Autodesk Inventor part; units mm, degrees
ref_plane "YZ Plane" through (0, 0, 0) normal (1, 0, 0) x (0, 1, 0)
ref_plane "XZ Plane" through (0, 0, 0) normal (0, 1, 0) x (-1, 0, 0)
ref_plane "XY Plane" through (0, 0, 0) normal (0, 0, 1) x (1, 0, 0)
sketch "Sketch1" plane through (0, 0, 0) normal (1, 0, 0) x (0, 1, 0)
  line L0 (4.2484, 4.9473) -> (-21.1516, 4.9473)
  line L1 (-21.1516, 4.9473) -> (-21.1516, -20.4527)
  line L2 (-21.1516, -20.4527) -> (4.2484, -20.4527)
  line L3 (4.2484, -20.4527) -> (4.2484, 4.9473)
  line L4 (1.0734, 1.7723) -> (-17.9766, 1.7723)
  line L5 (-17.9766, 1.7723) -> (-17.9766, -17.2777)
  line L6 (-17.9766, -17.2777) -> (1.0734, -17.2777)
  line L7 (1.0734, -17.2777) -> (1.0734, 1.7723)
  point P0 (0, 0)
  dimension "d0" = 25.4
  dimension "d1" = 25.4
  dimension "d2" = 3.175
extrude "Extrusion1" add sketch "Sketch1" along normal blind 381
sketch "Sketch2" plane through (0, -21.1516, -20.4527) normal (0, 0, -1) x (-1, 0, 0)
  line L0 (0, 0) -> (0, 25.4) construction
  line L1 (0, 12.7) -> (-12.7, 12.7) construction
  line L2 (-12.7, 12.7) -> (-38.1, 12.7) construction
  line L3 (-381, 0) -> (-381, 25.4) construction
  line L4 (-381, 12.7) -> (-368.3, 12.7) construction
  line L5 (-368.3, 12.7) -> (-342.9, 12.7) construction
  circle A0 centre (-368.3, 12.7) radius 2.5797
  circle A1 centre (-342.9, 12.7) radius 2.5797
  circle A2 centre (-12.7, 12.7) radius 2.5797
  circle A3 centre (-38.1, 12.7) radius 2.5797
  point P0 (0, 21.1516)
  dimension "d5" = 12.7
  dimension "d6" = 25.4
  dimension "d7" = 12.7
  dimension "d8" = 25.4
  dimension "d9" = 5.1594
  dimension "d10" = 5.1594
  dimension "d11" = 5.1594
  dimension "d12" = 5.1594
extrude "Extrusion2" cut sketch "Sketch2" against normal blind 431.8
properties part number "17in 1x1 Beam"
Input: part model. Units: mm. Frame: model coordinates. A direction names the side the tool comes from. Round coordinates to 2 decimals unless told otherwise and drop trailing zeros. Write each loop counter-clockwise with the first axis right and the second up, starting at its lowest first coordinate (ties: lowest second). Pieces come first, ordered by that corner, then holes.
1) Contact query for a flat-ended pin moving along its axis: P1, Ø4, axis at x = 342.9, y = -8.45, coming from the +Z side. Output: stop coordinate, or through.
2) Cut plane B-B (z = -2.25). Return the cut outline in (x, y).
3) Cut plane A-A (x = 109.5). Return the cut outline in (y, z), then the cut area to 3 significant figures.
4) Reachability of faces 4 (the flat face through (0, -20, -8)), 5 (the flat face through (188, -9, -17.278)) from +Z, -Z, +X, -X, +Y, -Y: full face, straight path, thin tool, end or side. Return the list, or none.
5) Draft query along Y for faces 1 (the flat face through (188, 1.073, -8)), 2 (the flat face through (188, -9, -20.453)), 3 (the flat face through (188, 4.248, -8)). Return one class per face: pulls with the +Y half, pulls with the -Y half, needs draft (parallel to the pull), parting line crosses it, or undercut.
6) Ray query, L1, parallel to X at y = -8.5, z = 3.5; L2, parallel to Z at x = 233.5, y = -11; L3, parallel to X at y = -6.5, z = -19. Return the intervals inside material, ascending.
Geometry says:
1. P1: passes through
2. outline: (0, -21.15) - (381, -21.15) - (381, -17.98) - (0, -17.98) - close; (0, 1.07) - (381, 1.07) - (381, 4.25) - (0, 4.25) - close
3. outline: (-21.15, -20.45) - (4.25, -20.45) - (4.25, 4.95) - (-21.15, 4.95) - close; hole (-17.98, -17.28) - (1.07, -17.28) - (1.07, 1.77) - (-17.98, 1.77) - close
3. area: 282 mm2
4. face 4: +Z, -Z, -X, +Y, -Y
4. face 5: +X, -X
5. face 1: undercut
5. face 2: needs draft
5. face 3: pulls with the +Y half
6. L1: x = 0 to 10.12, 15.28 to 35.52, 40.68 to 340.32, 345.48 to 365.72, 370.88 to 381
6. L2: z = -20.45 to -17.28, 1.77 to 4.95
6. L3: x = 0 to 11.01, 14.39 to 36.41, 39.79 to 341.21, 344.59 to 366.61, 369.99 to 381
